from build123d import *

# Parameters (mm, degrees)
SKETCH1_W           = 14.5
SKETCH1_H           = 15
BOSS_EXTRUDE1_DEPTH = 4.5
EXTRUDE_THIN1_DEPTH = 4.5
BOSS_EXTRUDE2_DEPTH = 9
FILLET2_R           = 0.5


with BuildPart() as part:
    # Sketch1 → Boss-Extrude1 (new body)
    with BuildSketch(Plane(origin=(0, 0, 0), x_dir=(1, 0, 0), z_dir=(0, 1, 0))):
        Rectangle(SKETCH1_W, SKETCH1_H)
    extrude(amount=BOSS_EXTRUDE1_DEPTH)

    # Sketch2 → Extrude-Thin1 (add)
    with BuildSketch(Plane(origin=(0, 4.5, 0), x_dir=(1, 0, 0), z_dir=(0, 1, 0))):
        with BuildLine():
            Line((-5.85, 5.540513031), (-5.85, 7.5))
            ThreePointArc((-5.85, 7.5), (-5.56028975, 8.318116508), (-4.820285198, 8.771591881))
            Line((-4.820285198, 8.771591881), (5.011361565, 10.861372913))
            ThreePointArc((5.011361565, 10.861372913), (7.149778281, 13.467770346), (5.078861565, 16.128115735))
            Line((5.078861565, 16.128115735), (-4.802785198, 18.494754348))
            ThreePointArc((-4.802785198, 18.494754348), (-5.799893246, 19.775661387), (-4.770285198, 21.030593485))
            Line((-4.770285198, 21.030593485), (5.061361565, 23.120374517))
            ThreePointArc((5.061361565, 23.120374517), (7.185209117, 26.043599889), (4.5, 28.461373039))
            Line((4.5, 28.461373039), (-6.14655289, 28.461373039))
            Line((-6.14655289, 28.461373039), (-6.14655289, 27.061373039))
            Line((-6.14655289, 27.061373039), (4.5, 27.061373039))
            ThreePointArc((4.5, 27.061373039), (5.792878464, 25.897260041), (4.770285198, 24.489781158))
            Line((4.770285198, 24.489781158), (-5.061361565, 22.400000126))
            ThreePointArc((-5.061361565, 22.400000126), (-7.199778281, 19.793602693), (-5.128861565, 17.133257304))
            Line((-5.128861565, 17.133257304), (4.752785198, 14.76661869))
            ThreePointArc((4.752785198, 14.76661869), (5.749893246, 13.485711651), (4.720285198, 12.230779554))
            Line((4.720285198, 12.230779554), (-5.111361565, 10.140998522))
            ThreePointArc((-5.111361565, 10.140998522), (-6.648294096, 9.199165056), (-7.25, 7.5))
            Line((-7.25, 7.5), (-7.25, 5.540513031))
            Line((-7.25, 5.540513031), (-5.85, 5.540513031))
        make_face()
    extrude(amount=-EXTRUDE_THIN1_DEPTH)

    # Sketch3 → Boss-Extrude2 (add)
    with BuildSketch(Plane(origin=(0, 4.5, 0), x_dir=(1, 0, 0), z_dir=(0, 1, 0))):
        with BuildLine():
            Line((1.4, 2.5), (1.4, -0.5))
            ThreePointArc((1.4, -0.5), (0, -1.9), (-1.4, -0.5))
            Line((-1.4, -0.5), (-1.4, 2.5))
            ThreePointArc((-1.4, 2.5), (0, 3.9), (1.4, 2.5))
        make_face()
    extrude(amount=BOSS_EXTRUDE2_DEPTH)

    # Fillet2
    fillet2_edges = [part.edges().sort_by_distance(p)[0] for p in [
        (0, 4.5, -3.9),
        (-1.4, 4.5, -1),
        (0, 4.5, 1.9),
        (1.4, 4.5, -1),
        (0, 13.5, -3.9),
        (-1.4, 13.5, -1),
        (0, 13.5, 1.9),
        (1.4, 13.5, -1),
    ]]
    fillet(fillet2_edges, radius=FILLET2_R)


solid = part.part
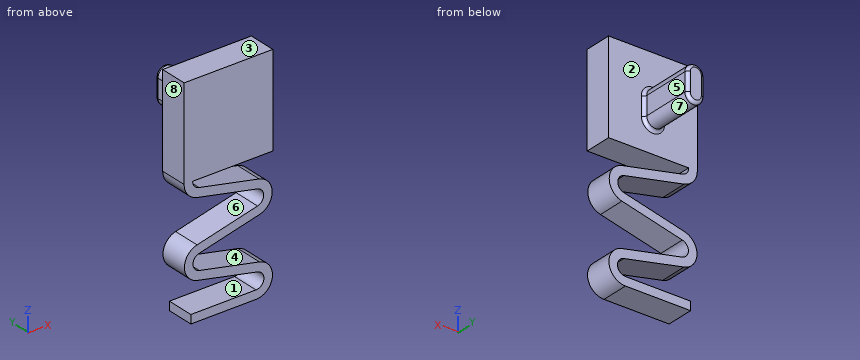
Geometry: final body of the model. Coordinates: model frame, mm. Face numbers are marked on the shaded views. A direction names the side the tool comes from. Coordinates: 2 decimals unless noted, no trailing zeros. Order: outer loops, then holes, each group sorted by start corner. A loop starts at its lowest first (then second) coordinate and runs counter-clockwise, first axis right, second up.
(1) Section query B-B (z = -2). Return the cut outline in (x, y), plus the area to 4 significant figures.
(2) Draft query along Z for the marked faces 1, 2 and 3. Return one class per face: pulls with the +Z half, pulls with the -Z half, needs draft (parallel to the pull), parting line crosses it, or undercut.
(3) Material intervals for probe 1 along Z at (x, y) = (-4.5, 4.25); probe 2 along Z at (x, y) = (-3, 3.5); probe 3 along X at (y, z) = (8.25, 0), sorted ascending.
(4) Section query A-A (x = 0). Return the cut outline in (y, z), plus the area to 3 significant figures.
(5) Access query for the marked faces 4, 5, 6, 7 and 8. Directions: +Z, -Z, +X, -X, +Y, -Y. A direction counts if a zero-diameter tool reaches every point of the face in a straight line with its end or side. Return the directions, or none.
(6) Section query C-C (y = 1.5). Return the cut outline in (x, z), plus the area to 3 significant figures.
(7) First-contact query: pin 1 (1.5 mm diameter, centred on y = 9.5, z = -1, fed in from -X); pin 2 (8 mm diameter, centred on x = 1, z = -24.5, fed in from +Y); pin 3 (2 mm diameter, centred on x = 1, y = 7.5, fed in from -Z). Flat tips, straight axial feed; report the tip coordinate or a pass-through.
(8) Section query D-D (x = -2.75). Return the cut outline in (y, z).
Solution:
1. outline: (-7.25, 0) - (7.25, 0) - (7.25, 4.5) - (1.9, 4.5) arc R0.5 cw to (1.4, 5) - (1.4, 13) arc R0.5 ccw to (0.9, 13.5) - (-0.9, 13.5) arc R0.5 ccw to (-1.4, 13) - (-1.4, 5) arc R0.5 cw to (-1.9, 4.5) - (-7.25, 4.5) - close
1. area: 90.45 mm2
2. face 1: undercut
2. face 2: needs draft
2. face 3: pulls with the +Z half
3. probe 1: z = -28.46 to -27.06, -22.52 to -21.09, -18.42 to -16.98, -10.27 to -8.84, -7.5 to 7.5
3. probe 2: z = -28.46 to -27.06, -22.84 to -21.41, -18.06 to -16.62, -10.59 to -9.16, -7.5 to 7.5
3. probe 3: x = -1.4 to 1.4
4. outline: (0, -28.46) - (4.5, -28.46) - (4.5, -27.06) - (0, -27.06) - close; (0, -23.48) - (4.5, -23.48) - (4.5, -22.04) - (0, -22.04) - close; (0, -17.34) - (4.5, -17.34) - (4.5, -15.9) - (0, -15.9) - close; (0, -11.23) - (4.5, -11.23) - (4.5, -9.8) - (0, -9.8) - close; (0, -7.5) - (4.5, -7.5) - (4.5, -4.4) arc R0.5 cw to (5, -3.9) - (13, -3.9) arc R0.5 ccw to (13.5, -3.4) - (13.5, 1.4) arc R0.5 ccw to (13, 1.9) - (5, 1.9) arc R0.5 cw to (4.5, 2.4) - (4.5, 7.5) - (0, 7.5) - close
4. area: 145 mm2
5. face 4: +X, +Y, -Y
5. face 5: +Z, -Z, +X, +Y
5. face 6: -X, +Y, -Y
5. face 7: -Z, +Y
5. face 8: +Z, -Z, -X, +Y, -Y
6. outline: (-7.25, -7.5) arc R2.7 ccw to (-5.11, -10.14) - (4.72, -12.23) arc R1.3 cw to (4.75, -14.77) - (-5.13, -17.13) arc R2.7 ccw to (-5.06, -22.4) - (4.77, -24.49) arc R1.3 cw to (4.5, -27.06) - (-6.15, -27.06) - (-6.15, -28.46) - (4.5, -28.46) arc R2.7 ccw to (5.06, -23.12) - (-4.77, -21.03) arc R1.3 cw to (-4.8, -18.49) - (5.08, -16.13) arc R2.7 ccw to (5.01, -10.86) - (-4.82, -8.77) arc R1.3 cw to (-5.85, -7.5) - (7.25, -7.5) - (7.25, 7.5) - (-7.25, 7.5) - close
6. area: 302 mm2
7. pin 1: stops at x = -1.4
7. pin 2: stops at y = 4.5
7. pin 3: stops at z = -3.9
8. outline: (0, -28.46) - (4.5, -28.46) - (4.5, -27.06) - (0, -27.06) - close; (0, -22.89) - (4.5, -22.89) - (4.5, -21.46) - (0, -21.46) - close; (0, -18) - (4.5, -18) - (4.5, -16.56) - (0, -16.56) - close; (0, -10.64) - (4.5, -10.64) - (4.5, -9.21) - (0, -9.21) - close; (0, -7.5) - (4.5, -7.5) - (4.5, 7.5) - (0, 7.5) - close
